from build123d import *

# Parameters (mm, degrees)
ENL_V_MAT_EXTRU_1_DEPTH = 158.508729917
ESQUISSE3_R             = 3.75
ENL_V_MAT_EXTRU_2_DEPTH = 158.508729917
ENL_V_MAT_EXTRU_3_DEPTH = 131.348301481


with BuildPart() as part:
    # Esquisse1 → Révolution1 (revolve)
    with BuildSketch(Plane.XY, mode=Mode.PRIVATE) as r_volution1_sk:
        with BuildLine():
            Line((0, 0), (29.566275292, 0))
            Line((29.566275292, 0), (29.566275292, 25))
            Line((29.566275292, 25), (10.566275292, 25))
            ThreePointArc((10.566275292, 25), (9.152061729, 25.585786438), (8.566275292, 27))
            Line((8.566275292, 27), (8.566275292, 40))
            Line((8.566275292, 40), (-22.933724708, 40))
            Line((-22.933724708, 40), (-25.433724708, 37.5))
            Line((-25.433724708, 37.5), (-62.433724708, 37.5))
            Line((-62.433724708, 37.5), (-64.933724708, 40))
            Line((-64.933724708, 40), (-96.433724708, 40))
            Line((-96.433724708, 40), (-96.433724708, 27))
            ThreePointArc((-96.433724708, 27), (-97.019511146, 25.585786438), (-98.433724708, 25))
            Line((-98.433724708, 25), (-117.433724708, 25))
            Line((-117.433724708, 25), (-117.433724708, 0))
            Line((-117.433724708, 0), (0, 0))
        make_face()
    revolve(r_volution1_sk.sketch.rotate(Axis((-130.768922499, 0, 0), (1, 0, 0)), 90), axis=Axis((-130.768922499, 0, 0), (1, 0, 0)))

    # Esquisse2 → Enlèv. mat.-Extru.1 (cut, through all)
    with BuildSketch(Plane.ZY.offset(117.433724708)):
        with BuildLine():
            Line((0, 7), (0, 0))
            Line((0, 0), (43.449782835, 0))
            Line((43.449782835, 0), (43.449782835, 44.497429883))
            Line((43.449782835, 44.497429883), (0, 44.497429883))
            Line((0, 44.497429883), (0, 13))
            ThreePointArc((0, 13), (3, 10), (0, 7))
        make_face()
        with BuildLine():
            Line((-12, 7), (0, 7))
            ThreePointArc((0, 7), (3, 10), (0, 13))
            Line((0, 13), (-12, 13))
            ThreePointArc((-12, 13), (-15, 10), (-12, 7))
        make_face()
    extrude(amount=-ENL_V_MAT_EXTRU_1_DEPTH, mode=Mode.SUBTRACT)

    # Esquisse3 → Enlèv. mat.-Extru.2 (cut, through all)
    with BuildSketch(Plane.ZY.offset(117.433724708)):
        with BuildLine():
            ThreePointArc((-9.252780862, 34.53184829), (-11.904431292, 29.939055022), (-7.311638024, 27.287404593))
            Line((-7.311638024, 27.287404593), (-9.252780862, 34.53184829))
        make_face()
        with BuildLine():
            Line((-9.252780862, 34.53184829), (-7.311638024, 27.287404593))
            ThreePointArc((-7.311638024, 27.287404593), (-5.307134417, 28.626771082), (-4.532209443, 30.909626441))
            ThreePointArc((-4.532209443, 30.909626441), (-5.999354084, 33.884701467), (-9.252780862, 34.53184829))
        make_face()
        with Locations((-22.627416998, 22.627416998)):
            Circle(ESQUISSE3_R)
        with Locations((-30.909626441, 8.282209443)):
            Circle(ESQUISSE3_R)
        with Locations((-30.909626441, -8.282209443)):
            Circle(ESQUISSE3_R)
        with Locations((-22.627416998, -22.627416998)):
            Circle(ESQUISSE3_R)
        with Locations((-8.282209443, -30.909626441)):
            Circle(ESQUISSE3_R)
        with Locations((8.282209443, -30.909626441)):
            Circle(ESQUISSE3_R)
        with Locations((22.627416998, -22.627416998)):
            Circle(ESQUISSE3_R)
        with Locations((30.909626441, -8.282209443)):
            Circle(ESQUISSE3_R)
    extrude(amount=-ENL_V_MAT_EXTRU_2_DEPTH, mode=Mode.SUBTRACT)

    # Esquisse4 → Enlèv. mat.-Extru.3 (cut, through all)
    with BuildSketch(Plane(origin=(0, 0, 0), x_dir=(1, 0, 0), z_dir=(0, 1, 0))):
        Polygon((8.566275292, -30.207539179), (2.377041681, -27.321452148), (2.377041681, -40), (8.566275292, -40), align=None)
        with BuildLine():
            Line((26.921370581, -25), (24.356829962, -10.45576741))
            ThreePointArc((24.356829962, -10.45576741), (11.303432421, -16.199399791), (2.377041681, -27.321452148))
            Line((2.377041681, -27.321452148), (8.566275292, -30.207539179))
            Line((8.566275292, -30.207539179), (8.566275292, -27))
            ThreePointArc((8.566275292, -27), (9.152061729, -25.585786438), (10.566275292, -25))
            Line((10.566275292, -25), (26.921370581, -25))
        make_face()
        with BuildLine():
            ThreePointArc((2.377041681, -27.321452148), (11.303432421, -16.199399791), (24.356829962, -10.45576741))
            Line((24.356829962, -10.45576741), (23.488589073, -5.531728645))
            ThreePointArc((23.488589073, -5.531728645), (8.259625276, -12.23263309), (-2.154497255, -25.208360839))
            Line((-2.154497255, -25.208360839), (2.377041681, -27.321452148))
        make_face()
        Polygon((29.566275292, -10.45576741), (24.356829962, -10.45576741), (26.921370581, -25), (29.566275292, -25), align=None)
    extrude(amount=-ENL_V_MAT_EXTRU_3_DEPTH, mode=Mode.SUBTRACT)


solid = part.part
Read the model definition and answer for the solid it produces. Units are mm, in the model's axes. A direction names the side the tool comes from. Round coordinates to 2 decimals unless told otherwise and drop trailing zeros. Use a Markdown table: item, result.
1) For a pull along X with two mould halves and no side action, classify faces 5 (the flat face through (-45, 7, -6)), 6 (the conical face through (-25.31, -27.47, -25.71)), 7 (the flat face through (2.377, -11, 34)), 8 (the conical face through (-62.59, -27.491, -25.734)) as pulls with the +X half, pulls with the -X half, needs draft (parallel to the pull), parting line crosses it, or undercut.
Answers follow:
| item | result |
|---|---|
| face 5 | needs draft |
| face 6 | undercut |
| face 7 | pulls with the +X half |
| face 8 | undercut |
2) The part is cut by section A-A (x = -77.5). Give the number of separate pieces and of enclosed holes in the cut face, plus the area to 3 significant figures.
Answers follow:
| item | result |
|---|---|
| separate pieces | 1 |
| enclosed holes | 9 |
| area | 3,290 mm2 |
3) A tool of negligible diameter and unlimited length cuts with its end or side. For faces 1 (the cylindrical face through (8.45, -14.57, 12.09)), 2 (the cylindrical face through (-108.067, -18.251, -17.085)), 3 (the flat face through (-45, 4, 0)), 4 (the flat face through (-45, 13, -6)), from which of +Z, -Z, +X, -X, +Y, -Y can it reach the whole face along a straight path? Write none if from no direction.
Answers follow:
| item | result |
|---|---|
| face 1 | +Y, -Y |
| face 2 | -X |
| face 3 | +Z, +X, -X, +Y |
| face 4 | +Z, +X, -X |
4) Straight lines are drawn through the part: line 1 along Y through (x, z) = (-86.5, -23); line 2 along Z through (x, y) = (0, -8); line 3 along Z through (x, y) = (-13, 24.5). For each, find the intervals that lie inside material, in ascending order. Write a range as [from, to].
Answers follow:
| item | result |
|---|---|
| line 1 | y = [-32.73, -26.36], [-18.9, 18.9], [26.36, 32.73] |
| line 2 | z = [-39.19, -34.65], [-27.17, 21.27], [26.21, 27.17], [34.65, 39.19] |
| line 3 | z = [-31.62, -25.88], [-19.38, 0] |
5) Flat-ended cylindrical pins translate along their axes: pin 1 (3.5 mm diameter, centred on x = -11.5, y = 4.5, fed in from +Z); pin 2 (3.5 mm diameter, centred on x = -17, z = -5, fed in from +Y); pin 3 (9.5 mm diameter, centred on x = -68.5, z = -5.5, fed in from -Y); pin 4 (7 mm diameter, centred on y = -8.28, z = 30.91, fed in from +X). Find the tip coordinate at first contact, or state that the pin passes through.
Answers follow:
| item | result |
|---|---|
| pin 1 | stops at z = 0 |
| pin 2 | stops at y = 39.87 |
| pin 3 | stops at y = -39.99 |
| pin 4 | passes through |
